from build123d import *

# Parameters (mm, degrees)
F0_W     = 6.86
F0_H     = 12.7
F1_DEPTH = 4.445
F2_R     = 3.175
F3_DEPTH = 8.89
F4_W     = 2.03
F4_H     = 0.75
F4_H_2   = 0.76
F5_DEPTH = 3.96


with BuildPart() as f1:
    # F0 (on Top) → F1 (new body, symmetric)
    with BuildSketch(Plane.XY):
        Rectangle(F0_W, F0_H)
    extrude(amount=F1_DEPTH, both=True)

    # F2 (on face) → F3 (join)
    with BuildSketch(Plane.XY.offset(4.445)):
        Circle(F2_R)
    extrude(amount=F3_DEPTH)

    # F4 (on face) → F5 (join)
    with BuildSketch(Plane(origin=(0, 0, -4.445), x_dir=(1, 0, 0), z_dir=(0, 0, -1))):
        Rectangle(F4_W, F4_H)
        with Locations((0, -4.7)):
            Rectangle(F4_W, F4_H_2)
        with Locations((0, 4.7)):
            Rectangle(F4_W, F4_H_2)
    extrude(amount=F5_DEPTH)

    # F6 (on Right) → F7 (revolve)
    with BuildSketch(Plane.YZ):
        with BuildLine():
            Line((-1.46, 22.275), (-1.46, 13.335))
            Line((-1.46, 13.335), (0, 13.335))
            Line((0, 13.335), (0, 23.735))
            ThreePointArc((0, 23.735), (-1.032376, 23.307376), (-1.46, 22.275))
        make_face()
    revolve(axis=Axis((0, 0, 18.535), (0, 0, -1)))


solid = f1.part
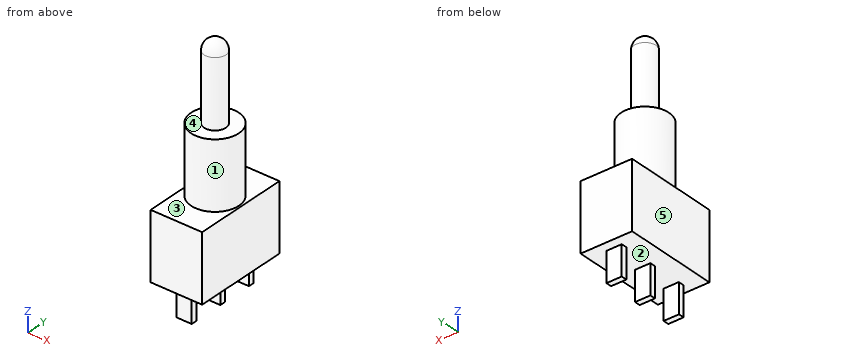
Check sheet for the modelled part. Datum: model origin and axes. Units: mm. Face numbers are marked on the shaded views. A direction names the side the tool comes from. Coordinates: 2 decimals unless noted, no trailing zeros. Loops run counter-clockwise (first coordinate to the right, second up) from the corner with the lowest first, then second, coordinate; pieces in that order, holes last. Notation, with made-up numbers: (25, 20.5) -> (44, 20.5) arc R20 ccw to (44, 44.5) -> close; hole circle Ø2 at (-14, 29.5). An arc over 180 degrees is marked (long way). Answer in a Markdown table with one row per item.
1. Sectioned sample at C-C, the plane z = 21.5. Record the boundary of the cut face in (x, y), then the cut area to 3 significant figures.
Check values:
| item | result |
|---|---|
| outline | circle Ø2.92 at (0, 0) |
| area | 6.70 mm2 |
2. Sectioned sample at D-D, the plane z = 8. Record the boundary of the cut face in (x, y) (3 decimals), then the cut area to 3 significant figures.
Check values:
| item | result |
|---|---|
| outline | circle Ø6.35 at (0, 0) |
| area | 31.7 mm2 |
3. Material ranges on line 1 along Z through (x, y) = (0.25, 3.75) (3 decimals); line 2 along Z through (x, y) = (1.5, -2.5) (3 decimals); line 3 along X through (y, z) = (0.25, -7) (3 decimals), recorded low to high. Write a range as [from, to].
Check values:
| item | result |
|---|---|
| line 1 | z = [-4.445, 4.445] |
| line 2 | z = [-4.445, 13.335] |
| line 3 | x = [-1.015, 1.015] |
4. Sectioned sample at B-B, the plane y = -2. Record the boundary of the cut face in (x, z) (3 decimals), then the cut area to 3 significant figures.
Check values:
| item | result |
|---|---|
| outline | (-3.43, -4.445) -> (3.43, -4.445) -> (3.43, 4.445) -> (2.466, 4.445) -> (2.466, 13.335) -> (-2.466, 13.335) -> (-2.466, 4.445) -> (-3.43, 4.445) -> close |
| area | 105 mm2 |
5. Release check for a two-part mould opening along Y. For the marked faces 1, 2 and 3 record: released by +Y, released by -Y, zero draft, split by the parting line, or undercut.
Check values:
| item | result |
|---|---|
| face 1 | split by the parting line |
| face 2 | undercut |
| face 3 | zero draft |
6. Go/stop test with flat-tipped pins: pin 1 (0.8 mm diameter, centred on y = 0, z = -7.5, fed in from +X) (3 decimals); pin 2 (1 mm diameter, centred on x = 0, z = -7, fed in from +Y); pin 3 (1 mm diameter, centred on x = 0, z = -6.5, fed in from -Y); pin 4 (3.5 mm diameter, centred on x = 0, y = 3, fed in from -Z) (3 decimals). Record where each tip stops, or that it passes through.
Check values:
| item | result |
|---|---|
| pin 1 | stops at x = 1.015 |
| pin 2 | stops at y = 5.08 |
| pin 3 | stops at y = -5.08 |
| pin 4 | stops at z = -8.405 |
7. Access from +Z, -Z, +X, -X, +Y, -Y to the whole of each face (thin tool, end or side, straight path). Record for the marked faces 4 and 5.
Check values:
| item | result |
|---|---|
| face 4 | +Z |
| face 5 | +Z, -Z, -X, +Y, -Y |
8. Sectioned sample at A-A, the plane x = 2.5. Record the boundary of the cut face in (y, z) (3 decimals).
Check values:
| item | result |
|---|---|
| outline | (-6.35, -4.445) -> (6.35, -4.445) -> (6.35, 4.445) -> (1.957, 4.445) -> (1.957, 13.335) -> (-1.957, 13.335) -> (-1.957, 4.445) -> (-6.35, 4.445) -> close |
